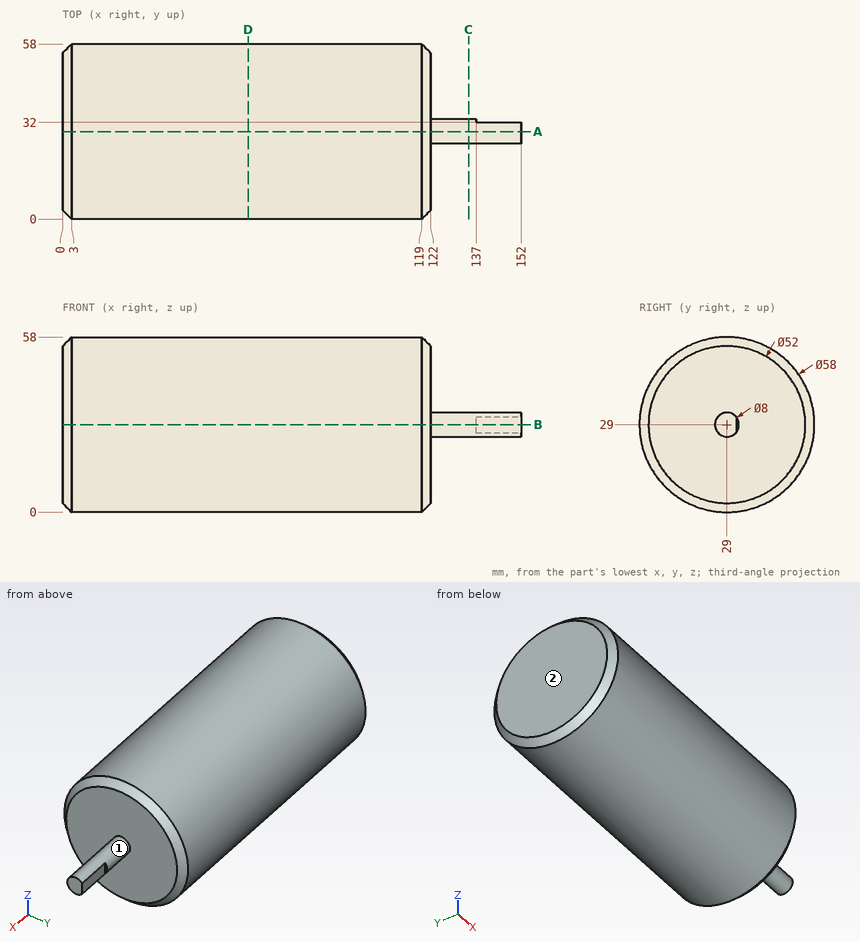
For this review, use the dimensioned drawing (mm, ordinates from the lowest corner) and the shaded views. A direction names the side the tool comes from. Coordinates: 2 decimals unless noted, no trailing zeros. Order: outer loops, then holes, each group sorted by start corner. A loop starts at its lowest first (then second) coordinate and runs counter-clockwise, first axis right, second up. Notation, with made-up numbers: (33.5, 1) - (57.5, 1) arc R28 cw to (57.5, 23) - close; hole circle Ø11 at (-23, 73). An arc over 180 degrees is marked (long way). Use one line per item in the form item = value.
Q1. For probe 1 along X at (y, z) = (45, 36); probe 2 along Y at (x, z) = (98, 29); probe 3 along Z at (x, y) = (51, 49), list the stretches that pass through material, from the lowest coordinate up. Write a range as from..to.
Checked values:
probe_1 = 0..122
probe_2 = 0..58
probe_3 = 8..50
Q2. Consider section D-D (x = 61.5). Give the boundary of the cut face in (y, z).
Checked values:
outline = circle Ø58 at (29, 29)
Q3. For P1, Ø6, axis at y = 13.5, z = 8, coming from the +X side; P2, Ø3, axis at x = 62.5, y = 8, coming from the +Z side; P3, Ø5, axis at x = 70, z = 43.5, coming from the -Y side, all flat-tipped, find the tip position at first contact; note any pin that passes through.
Checked values:
P1 = 122
P2 = 50.47
P3 = 2.6
Q4. Consider section C-C (x = 134.5). Give the boundary of the cut face in (y, z).
Checked values:
outline = circle Ø8 at (29, 29)
Q5. Consider section A-A (y = 29). Give the boundary of the cut face in (x, z).
Checked values:
outline = (0, 3) - (3, 0) - (119, 0) - (122, 3) - (122, 25) - (152, 25) - (152, 33) - (122, 33) - (122, 55) - (119, 58) - (3, 58) - (0, 55) - close
Q6. Consider section B-B (z = 29). Give the boundary of the cut face in (x, y).
Checked values:
outline = (0, 3) - (3, 0) - (119, 0) - (122, 3) - (122, 25) - (152, 25) - (152, 32) - (137, 32) - (137, 33) - (122, 33) - (122, 55) - (119, 58) - (3, 58) - (0, 55) - close
Q7. For the marked faces 1 and 2, list the 3-axis set-ups (+Z, -Z, +X, -X, +Y, -Y) from which the entire face can be reached by the end or side of a thin tool; tool diameter is ignored.
Checked values:
face_1 = +X
face_2 = +Z, -Z, -X, +Y, -Y
